Part print with two shaded views. Sizes in mm from the minimum x, y, z corner. Round coordinates to 2 decimals unless told otherwise and drop trailing zeros. Loops run counter-clockwise (first coordinate to the right, second up) from the corner with the lowest first, then second, coordinate; pieces in that order, holes last. Notation, with made-up numbers: M 65.5,-22.5 L 78.5,-22.5 A24 cw 78.5,12.5 Z; hole C 26,-7 d1. An arc over 180 degrees is marked long. Use a Markdown table: item, result. Add a question column.
Item 1: Pin check, flat tips, straight feed: P1, Ø0.9, axis at y = 2, z = 2, coming from the -X side; P2, Ø1.5, axis at x = 52.5, z = 2, coming from the +Y side. Stop position of each tip, or through.
Item 2: Saw through at A-A on z = 1.95. Write the cut outline in (x, y), then the cut area to 3 significant figures.
Item 3: Saw through at B-B on y = 113. Write the cut outline in (x, z).
Item 4: Saw through at C-C on x = 50.5. Write the cut outline in (y, z).
Item 5: Wall check: L1, parallel to Y at x = 61, z = 2.65; L2, parallel to X at y = 108.5, z = 1; L3, parallel to X at y = 83.5, z = 1.45. Give the ranges that are in metal, low to high. Write a range as from..to.
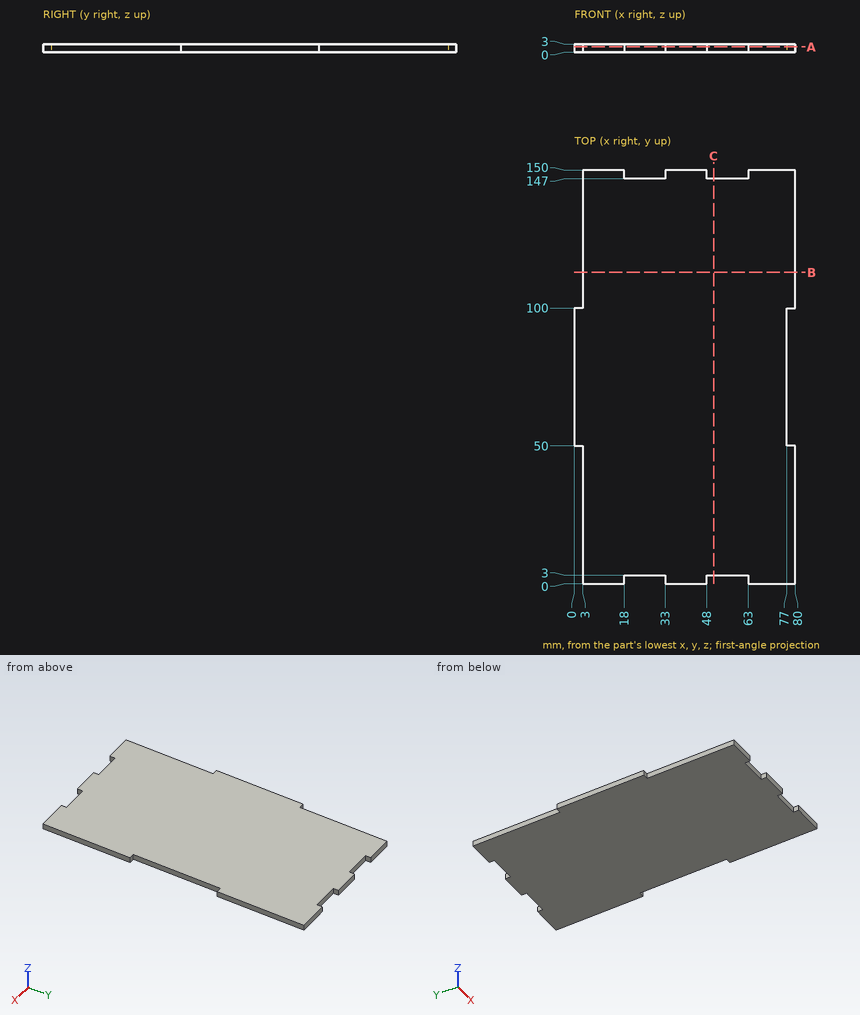
Entries:
| question | item | result |
|---|---|---|
| 1 | P1 | x = 3 |
| 1 | P2 | y = 147 |
| 2 | outline | M 0,50 L 3,50 L 3,0 L 18,0 L 18,3 L 33,3 L 33,0 L 48,0 L 48,3 L 63,3 L 63,0 L 80,0 L 80,50 L 77,50 L 77,100 L 80,100 L 80,150 L 63,150 L 63,147 L 48,147 L 48,150 L 33,150 L 33,147 L 18,147 L 18,150 L 3,150 L 3,100 L 0,100 Z |
| 2 | area | 11,400 mm2 |
| 3 | outline | M 3,0 L 80,0 L 80,3 L 3,3 Z |
| 4 | outline | M 3,0 L 147,0 L 147,3 L 3,3 Z |
| 5 | L1 | 3..147 |
| 5 | L2 | 3..80 |
| 5 | L3 | 0..77 |
